Geometry: final body of the model. Coordinates: model frame, mm. Face numbers are marked on the shaded views. A direction names the side the tool comes from. Coordinates: 2 decimals unless noted, no trailing zeros. Write each loop counter-clockwise with the first axis right and the second up, starting at its lowest first coordinate (ties: lowest second). Pieces come first, ordered by that corner, then holes. Notation, with made-up numbers: M 54.25,32 L 113.25,32 A27 ccw 113.25,57 Z; hole C -16.5,49 d4. An arc over 180 degrees is marked long. Write item = value, one per line. Start each with the question number.
Item 1: Reachability of the marked faces 1 and 2 from +Z, -Z, +X, -X, +Y, -Y: full face, straight path, thin tool, end or side. Return the list, or none.
Item 2: Section B-B on x = 17. Output: boundary loops of the cut face in (y, z).
Item 3: First-contact query: pin 1 Ø6 at (x, y) = (31.5, -5.5) entering from +Z; pin 2 Ø0.6 at (y, z) = (-33.5, 93) entering from -X; pin 3 Ø10 at (y, z) = (-10.5, 56.5) entering from +X. Flat tips, straight axial feed; report the tip coordinate or a pass-through.
Item 4: Pull-direction query (X, two-part tool) for the marked faces 3, 4 and 5; classes: +X half, -X half, draft (parallel to the pull), parting line (faces both ways), or undercut.
Item 5: Section A-A on z = 23. Output: boundary loops of the cut face in (x, y).
Item 6: Ray query, L1, parallel to Y at x = -2, z = 14.5; L2, parallel to Y at x = -23.5, z = 11.5; L3, parallel to X at y = 30.5, z = 14. Return the intervals inside material, ascending. Write a range as [from, to].
Item 7: Section C-C on y = 25.5. Output: boundary loops of the cut face in (x, z), plus the area to 3 significant figures.
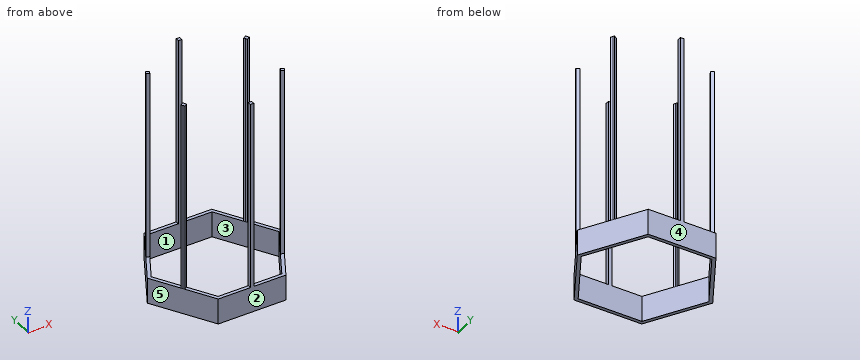
from build123d import *

# Parameters (mm, degrees)
F1_DEPTH = 15
F2_W     = 1
F2_H     = 2
F3_DEPTH = 110
F4_W     = 2
F4_H     = 2
F5_DEPTH = 2


with BuildPart() as f1:
    # F0 (on Top) → F1 (new body)
    with BuildSketch(Plane.XY):
        Polygon((-19.918584, -34.5), (19.918584, -34.5), (39.837169, 0), (19.918584, 34.5), (-19.918584, 34.5), (-39.837169, 0), align=None)
        Polygon((37.527767, 0), (18.763884, -32.5), (-18.763884, -32.5), (-37.527767, 0), (-18.763884, 32.5), (18.763884, 32.5), align=None, mode=Mode.SUBTRACT)
    extrude(amount=F1_DEPTH)

    # F2 (on face) → F3 (join)
    with BuildSketch(Plane.XY.offset(15)):
        Polygon((-28.645826, 15.383975), (-28.145826, 16.25), (-29.877876, 17.25), (-30.377876, 16.383975), align=None)
        Polygon((-29.877876, 17.25), (-28.145826, 16.25), (-27.645826, 17.116025), (-29.377876, 18.116025), align=None)
        with Locations((-0.5, 33.5)):
            Rectangle(F2_W, F2_H)
        with Locations((0.5, 33.5)):
            Rectangle(F2_W, F2_H)
        Polygon((27.645826, 17.116025), (28.145826, 16.25), (29.877876, 17.25), (29.377876, 18.116025), align=None)
        Polygon((29.877876, 17.25), (28.145826, 16.25), (28.723176, 15.25), (30.455227, 16.25), align=None)
        Polygon((28.145826, -16.25), (29.877876, -17.25), (30.377876, -16.383975), (28.645826, -15.383975), align=None)
        Polygon((27.645826, -17.116025), (29.377876, -18.116025), (29.877876, -17.25), (28.145826, -16.25), align=None)
        with Locations((0.5, -33.5)):
            Rectangle(F2_W, F2_H)
        with Locations((-0.5, -33.5)):
            Rectangle(F2_W, F2_H)
        Polygon((-29.877876, -17.25), (-29.300526, -18.25), (-27.568475, -17.25), (-28.145826, -16.25), align=None)
        Polygon((-30.377876, -16.383975), (-29.877876, -17.25), (-28.145826, -16.25), (-28.645826, -15.383975), align=None)
    extrude(amount=F3_DEPTH)

    # F4 (on face) → F5 (join)
    with BuildSketch(Plane(origin=(0, 34.5, 0), x_dir=(-1, 0, 0), z_dir=(0, 1, 0))):
        with Locations((0, 36)):
            Rectangle(F4_W, F4_H)
    extrude(amount=-F5_DEPTH)


solid = f1.part
Responses:
q1.face_1 = +Z, -Z
q1.face_2 = +Z, -Z, +X, -X, -Y
q2.outline = M -34.5,0 L -32.5,0 L -32.5,15 L -34.5,15 Z; M 32.5,0 L 34.5,0 L 34.5,15 L 32.5,15 Z
q3.pin_1 = 15
q3.pin_2 = -1
q3.pin_3 = 28.85
q4.face_3 = undercut
q4.face_4 = draft
q4.face_5 = -X half
q5.outline = M -30.38,-16.38 L -29.88,-17.25 L -29.3,-18.25 L -27.57,-17.25 L -28.15,-16.25 L -28.65,-15.38 Z; M -30.38,16.38 L -28.65,15.38 L -27.65,17.12 L -29.38,18.12 Z; M -1,-34.5 L 1,-34.5 L 1,-32.5 L -1,-32.5 Z; M -1,32.5 L 1,32.5 L 1,34.5 L -1,34.5 Z; M 27.65,-17.12 L 29.38,-18.12 L 30.38,-16.38 L 28.65,-15.38 Z; M 27.65,17.12 L 28.15,16.25 L 28.72,15.25 L 30.46,16.25 L 29.88,17.25 L 29.38,18.12 Z
q6.L1 = [-34.5, -32.5], [32.5, 34.5]
q6.L2 = [-28.3, -24.3], [24.3, 28.3]
q6.L3 = [-22.23, -19.92], [19.92, 22.23]
q7.outline = M -25.11,0 L -22.81,0 L -22.81,15 L -25.11,15 Z; M 22.81,0 L 25.11,0 L 25.11,15 L 22.81,15 Z
q7.area = 69.3 mm²
